Geometry check sheet. Reference: the model listing, model coordinates, mm. Round coordinates to 2 decimals unless told otherwise and drop trailing zeros. Write each loop counter-clockwise with the first axis right and the second up, starting at its lowest first coordinate (ties: lowest second). Pieces come first, ordered by that corner, then holes. Notation, with made-up numbers: M 45,74 L 70,74 A12 cw 70,90 Z; hole C 9,-13 d5. An arc over 180 degrees is marked long. Put each result on its own line as item: value. Start each with the question number.
(1) Section check C-C on x = 0. Record the cut outline in (y, z).
(2) Section check A-A on z = -8.5. Record the cut outline in (x, y).
(3) Section check B-B on y = 1.5. Record the cut outline in (x, z).
(4) Gauge pin test, flat end, axial feed: pin 1 (1.1 mm diameter, centred on y = 1.5, z = -8.5, fed in from -X). Record the tip position at first contact, or that the pin passes through.
(5) Material ranges on probe 1 along Z at (x, y) = (0, 1.5); probe 2 along Y at (x, z) = (0, -5); probe 3 along Y at (x, z) = (0, -8.75), recorded low to high.
Autodesk Inventor part; units mm, degrees
ref_plane "YZ Plane" through (0, 0, 0) normal (1, 0, 0) x (0, 1, 0)
ref_plane "XZ Plane" through (0, 0, 0) normal (0, 1, 0) x (-1, 0, 0)
ref_plane "XY Plane" through (0, 0, 0) normal (0, 0, 1) x (1, 0, 0)
sketch "Sketch1" plane through (0, 0, 0) normal (0, 1, 0) x (-1, 0, 0)
  line L0 (0, 0) -> (0, -12) construction
  line L1 (-0.1, 0) -> (-0.1, -12)
  line L2 (0.1, -12) -> (0.1, 0)
  arc A0 (0.1, 0) -> (-0.1, 0) centre (0, 0) ccw
  arc A1 (-0.1, -12) -> (0.1, -12) centre (0, -12) ccw
  point P0 (0, -6)
  dimension "d0" = 12
  dimension "d1" = 0.2
extrude "Extrusion1" add sketch "Sketch1" along normal blind 3
sketch "Sketch2" plane through (0.1, 0, 0) normal (1, 0, 0) x (0, 0, -1)
  line L0 (12.1, 0) -> (12.1, 3)
  line L1 (12.1, 1.5) -> (10.1, 1.5)
  circle A0 centre (10.1, 1.5) radius 0.6
  point P0 (0, 0)
  dimension "d4" = 2
  dimension "d5" = 1.2
extrude "Extrusion2" cut sketch "Sketch2" against normal blind 3
sketch "Sketch3" plane through (0.1, 0, 0) normal (1, 0, 0) x (0, 0, -1)
  line L0 (0, 0) -> (0, 3)
  line L1 (0, 1.5) -> (5, 1.5)
  line L2 (5, 1.5) -> (8.5, 1.5)
  circle A0 centre (5, 1.5) radius 0.6
  circle A1 centre (8.5, 1.5) radius 0.6
  dimension "d8" = 5
  dimension "d9" = 3.5
  dimension "d10" = 1.2
  dimension "d11" = 1.2
extrude "Extrusion3" cut sketch "Sketch3" against normal blind 10
sketch "Sketch4" plane through (-0.1, 0, -12) normal (-1, 0, 0) x (0, 0, 1)
  circle A0 centre (3.5, 1.5) radius 0.6
  circle A1 centre (7, 1.5) radius 0.6
  circle A2 centre (1.9, 1.5) radius 0.6
  line L0 (0, 0) -> (12, 0)
  line L1 (12, 0) -> (12, 3)
  line L2 (0, 3) -> (12, 3)
  line L3 (0, 0) -> (0, 3)
  line L4 (0, 0) -> (0, 3)
  line L5 (0, 3) -> (12, 3)
  line L6 (0, 0) -> (2.5, 0)
  line L7 (2.5, 0) -> (2.5, 3)
  line L8 (2.5, 3) -> (0, 3)
  line L9 (0, 3) -> (0, 0)
  line L10 (0, 0) -> (-0.8, 0)
  line L11 (-0.8, 0) -> (-0.8, 3)
  line L12 (-0.8, 3) -> (0, 3)
  line L13 (0, 3) -> (0, 0)
  point P0 (2.5, 1.5)
  point P1 (2.5, 3)
  dimension "d14" = 2.5
  dimension "d15" = 0.8
  dimension "d16" = 3
extrude "Extrusion4" cut sketch "Sketch4" against normal blind 10 contours L7 L0 L3 L2 | L10 L11 L12 L3
properties part number "fin_12mm_h"
Answers follow:
1. outline: M 0,-9.5 L 3,-9.5 L 3,0.1 L 0,0.1 Z; hole C 1.5,-8.5 d1.2; hole C 1.5,-5 d1.2
2. outline: M -0.1,0 L 0.1,0 L 0.1,0.9 L -0.1,0.9 Z; M -0.1,2.1 L 0.1,2.1 L 0.1,3 L -0.1,3 Z
3. outline: M -0.1,-9.5 L 0.1,-9.5 L 0.1,-9.1 L -0.1,-9.1 Z; M -0.1,-7.9 L 0.1,-7.9 L 0.1,-5.6 L -0.1,-5.6 Z; M -0.1,-4.4 L 0.1,-4.4 L 0.1,0 A0.1 ccw -0.1,0 Z
4. pin 1: passes through
5. probe 1: z = -9.5 to -9.1, -7.9 to -5.6, -4.4 to 0.1
5. probe 2: y = 0 to 0.9, 2.1 to 3
5. probe 3: y = 0 to 0.95, 2.05 to 3
